Autodesk Fusion 360 part; units mm, degrees
sketch "Sketch1" plane through (0, 0, 0) normal (0, 0, 1) x (1, 0, 0)
  line L0 (36, 27) -> (-36, 27)
  line L1 (-36, 27) -> (-36, -27)
  line L2 (-36, -27) -> (36, -27)
  line L3 (36, -27) -> (36, 27)
  line L4 (36, 30.6) -> (-36, 30.6)
  line L5 (-36, 35.6) -> (-36, -30.6)
  line L6 (-36, -30.6) -> (36, -30.6)
  line L7 (36, -30.6) -> (36, 30.6)
  line L8 (33, 35.6) -> (-36, 35.6)
  line L9 (41, -27.6) -> (41, 27.6)
  line L10 (33, -35.6) -> (-36, -35.6)
  line L11 (-36, -35.6) -> (-36, 30.6)
  arc A0 (41, 27.6) -> (33, 35.6) centre (33, 27.6) ccw
  arc A1 (33, -35.6) -> (41, -27.6) centre (33, -27.6) ccw
  circle A2 centre (-31, 0) radius 1.75
  line L12 (-31, 11) -> (-10, 11)
  arc A3 (-10, 11) -> (-10, 19) centre (-10, 15) ccw
  line L13 (-10, 19) -> (-31, 19)
  arc A4 (-31, 19) -> (-31, 11) centre (-31, 15) ccw
  line L14 (-31, 15) -> (-10, 15) construction
  line L15 (1.75, 0) -> (22.5, 0)
  line L16 (-31, -11) -> (-10, -11)
  line L17 (-10, -19) -> (-31, -19)
  arc A5 (-10, -19) -> (-10, -11) centre (-10, -15) ccw
  arc A6 (-31, -11) -> (-31, -19) centre (-31, -15) ccw
  circle A7 centre (-10, 0) radius 1.75
  dimension "d1" = 72
  dimension "d2" = 54
  dimension "d3" = 61.2
  dimension "d6" = 8
  dimension "d32" = 3.5
  dimension "d34" = 8
  dimension "d40" = 3.5
extrude "Extrude1" add sketch "Sketch1" along normal blind 6.15 contours L3 L4 L5 L6 L7 L8 L9 L10 L11 A0 A1 | L0 L4 L5 L7 L11 | L2 L5 L6 L7 L11
extrude "Extrude2" add sketch "Sketch1" along normal blind 24 contours L3 L4 L5 L6 L7 L8 L9 L10 L11 A0 A1
extrude "Extrude3" add sketch "Sketch1" along normal blind 27 and the other way blind -24
sketch "Sketch2" plane through (0, -35.6, 0) normal (0, -1, 0) x (1, 0, 0)
  line L0 (-36, 0) -> (33, 0)
  line L1 (33, 0) -> (33, 27)
  line L2 (-36, 27) -> (-36, 0)
  line L3 (-36, 0) -> (-49.5029, 27)
  line L4 (-36, 0) -> (-6, 0) construction
  line L5 (-36, 27) -> (-49.5029, 27)
  line L6 (33, 27) -> (-36, 27)
  line L7 (-36, 27) -> (-36, 24)
  line L8 (-36, 24) -> (-36.4845, 24)
  line L9 (-36.4845, 24) -> (-48.0026, 24)
  line L10 (-36, 0) -> (-36, 6.4)
  line L11 (-36, 6.4) -> (-36, 6)
  line L12 (-36, 6.4) -> (-39.2007, 6.4)
  line L13 (-36, 0) -> (-32.4, 0)
  line L14 (-49.5029, 27) -> (-47.5029, 27)
  line L15 (-36, 6.4) -> (-32.4, 6.4)
  line L16 (-32.4, 6.4) -> (-32.4, 0)
  dimension "d11" = 116.57
  dimension "d25" = 6.4
  dimension "d36" = 3.6
  dimension "d37" = 2
extrude "Extrude4" add sketch "Sketch2" against normal blind 5 contours L2 L3 L10 L11 L12 | L2 L3 L8 L9 L12
extrude "Extrude5" add sketch "Sketch2" along normal blind -71.2 and the other way blind 66.2 contours L2 L3 L10 L11 L12 | L2 L3 L8 L9 L12
extrude "Extrude6" add sketch "Sketch2" against normal blind 71.2 contours L2 L3 L5 L7 L8 L9 L14
extrude "Extrude7" cut sketch "Sketch2" along normal blind -8.6 and the other way blind 5 contours L0 L2 L10 L11 L13 L15 L16
extrude "Extrude8" cut sketch "Sketch2" along normal blind -66.2 and the other way blind 62.6 contours L0 L2 L10 L11 L13 L15 L16
chamfer "Chamfer2" distance 1 angle 45 2 edges at (-32.6316, 0.6328, 24) (-11.6316, 0.6328, 24)
sketch "Sketch3" plane through (0, 0, 27) normal (0, 0, 1) x (-1, 0, 0)
  arc A0 (10, 19) -> (10, 11) centre (10, 15) ccw
  line L0 (10, 19) -> (31, 19)
  arc A1 (31, 11) -> (31, 19) centre (31, 15) ccw
  line L1 (31, 11) -> (10, 11)
  circle A2 centre (31, 0) radius 1.75
  circle A3 centre (10, 0) radius 1.75
  arc A4 (31, -19) -> (31, -11) centre (31, -15) ccw
  line L2 (31, -19) -> (10, -19)
  arc A5 (10, -11) -> (10, -19) centre (10, -15) ccw
  line L3 (10, -11) -> (31, -11)
  line L4 (49.5029, 35.6) -> (-33, 35.6)
  arc A6 (-33, 35.6) -> (-41, 27.6) centre (-33, 27.6) ccw
  line L5 (-41, 27.6) -> (-41, -27.6)
  arc A7 (-41, -27.6) -> (-33, -35.6) centre (-33, -27.6) ccw
  line L6 (-33, -35.6) -> (49.5029, -35.6)
  line L7 (49.5029, -35.6) -> (49.5029, 35.6)
  line L8 (2.0837, -40) -> (-45, -40)
  line L9 (-45, -40) -> (-45, 40)
  line L10 (-45, 40) -> (2.0837, 40)
  line L11 (2.0837, 40) -> (2.0837, -40)
extrude "Extrude9" cut sketch "Sketch3" against normal blind 55 contours L4 A6 L5 A7 L6 L11 | L4 A6 L5 A7 L6 L8 L9 L10 L11
chamfer "Chamfer3" distance 1 angle 45 2 edges at (-32.4, -28.8, 6.15) (-32.4, 28.8, 6.15)
Part model, mm, in its own coordinate system. A direction names the side the tool comes from. Give positions to 0.01 mm unless a question says otherwise; leave off trailing zeros. Loops run counter-clockwise (first coordinate to the right, second up) from the corner with the lowest first, then second, coordinate; pieces in that order, holes last. Notation, with made-up numbers: M -28,59 L 19,59 A14 ccw 19,71 Z; hole C 86,50 d2. An arc over 180 degrees is marked long. Return JSON: item names as keys, results as strings.
1) Flat gauge pins, fed straight in: pin 1 Ø1.8 at (y, z) = (29.5, 3) entering from -X; pin 2 Ø4.5 at (x, y) = (-10, 0) entering from -Z; pin 3 Ø5 at (x, y) = (-25.5, 20.5) entering from -Z. Where does each tip first touch, or does it go through?
Calculated:
{"pin 1": "stops at x = -32.4", "pin 2": "stops at z = 24.5", "pin 3": "stops at z = 24"}
2) Saw through at A-A, the plane x = -18.5. List the corners of the cut face in (y, z).
Calculated:
{"outline": "M -35.6,0 L -27,0 L -27,6.15 L -30.6,6.15 L -30.6,24 L -19,24 L -19,27 L -35.6,27 Z; M -11,24 L 11,24 L 11,27 L -11,27 Z; M 19,24 L 30.6,24 L 30.6,6.15 L 27,6.15 L 27,0 L 35.6,0 L 35.6,27 L 19,27 Z"}
3) Drill centre lines: line 1 (Y direction, x = -31, z = 26.55); line 2 (Y direction, x = -26.5, z = 10.25); line 3 (Z direction, x = -12, y = -30). Where is each one in solid material? Low to high.
Calculated:
{"line 1": "y = -35.6 to -19, -11 to -1.75, 1.75 to 11, 19 to 35.6", "line 2": "y = -35.6 to -30.6, 30.6 to 35.6", "line 3": "z = 0 to 6.15, 24 to 27"}
4) 3-axis set-ups, long thin cutter, end or side, ignore diameter. For faces 4 (the face through (-17, 27, 3)), 5 (the face through (-21, -11, 25)), 6 (the face through (-19, -31, 0)), 7 (the face through (-32.4, -29, 3)): which of +Z, -Z, +X, -X, +Y, -Y reach the whole face in a straight line?
Calculated:
{"face 4": "-Z, +X, -X", "face 5": "+Z, -Z", "face 6": "-Z, +X, -X, +Y, -Y", "face 7": "-Z, -X"}
5) Saw through at B-B, the plane y = -15. List the corners of the cut face in (x, z).
Calculated:
{"outline": "M -49.5,27 L -48,24 L -35,24 L -35,27 Z; M -6,24 L -2.08,24 L -2.08,27 L -6,27 Z"}
6) Pull direction X, two halves, no side cores. Call faces 1 (the face through (-8.331, -0.526, 25.986)), 2 (the face through (-48.221, -2.803, 24.437)), 3 (the face through (-25, 30.6, 15)): released by +X, released by -X, zero draft, split by the parting line, or undercut.
Calculated:
{"face 1": "undercut", "face 2": "released by -X", "face 3": "zero draft"}
7) Saw through at D-D, the plane y = 0. List the corners of the cut face in (x, z), then the cut area to 3 significant figures.
Calculated:
{"outline": "M -49.5,27 L -48,24 L -33.75,24 L -32.75,25 L -32.75,27 Z; M -29.25,25 L -28.25,24 L -12.75,24 L -11.75,25 L -11.75,27 L -29.25,27 Z; M -8.25,25 L -7.25,24 L -2.08,24 L -2.08,27 L -8.25,27 Z", "area": "117 mm2"}
8) Saw through at C-C, the plane z = 19.25. List the corners of the cut face in (x, y), then the cut area to 3 significant figures.
Calculated:
{"outline": "M -45.63,-35.6 L -2.08,-35.6 L -2.08,-30.6 L -45.63,-30.6 Z; M -45.63,30.6 L -2.08,30.6 L -2.08,35.6 L -45.63,35.6 Z", "area": "435 mm2"}
